from build123d import *

# Parameters (mm, degrees)
SKETCH1_R           = 10
BOSS_EXTRUDE1_DEPTH = 5
BOSS_EXTRUDE3_START = 2
SKETCH3_R           = 12.5
SKETCH3_R_2         = 3.5
SKETCH3_R_3         = 0.95
BOSS_EXTRUDE3_DEPTH = 2


with BuildPart() as part:
    # Sketch1 → Boss-Extrude1 (new body)
    with BuildSketch(Plane.XY):
        with BuildLine():
            Line((-25, 13.756613757), (-25, 11.243386243))
            Line((-25, 11.243386243), (-22.480898871, 11.243386243))
            ThreePointArc((-22.480898871, 11.243386243), (-15.409831059, 8.314454055), (-12.480898871, 1.243386243))
            Line((-12.480898871, 1.243386243), (-12.480898871, 0.690770135))
            ThreePointArc((-12.480898871, 0.690770135), (0, -12.5), (12.480898871, 0.690770135))
            Line((12.480898871, 0.690770135), (12.480898871, 1.243386243))
            ThreePointArc((12.480898871, 1.243386243), (15.409831059, 8.314454055), (22.480898871, 11.243386243))
            Line((22.480898871, 11.243386243), (25, 11.243386243))
            Line((25, 11.243386243), (25, 13.756613757))
            Line((25, 13.756613757), (-25, 13.756613757))
        make_face()
        Circle(SKETCH1_R, mode=Mode.SUBTRACT)
    extrude(amount=BOSS_EXTRUDE1_DEPTH)

    # Sketch3 → Boss-Extrude3 (add)
    with BuildSketch(Plane(origin=(0, 0, 0), x_dir=(-1, 0, 0), z_dir=(0, 0, -1)).offset(BOSS_EXTRUDE3_START)):
        Circle(SKETCH3_R)
        Circle(SKETCH3_R_2, mode=Mode.SUBTRACT)
        with Locations((7.5, 0)):
            Circle(SKETCH3_R_3, mode=Mode.SUBTRACT)
        with Locations((-7.5, 0)):
            Circle(SKETCH3_R_3, mode=Mode.SUBTRACT)
    extrude(amount=-BOSS_EXTRUDE3_DEPTH)


solid = part.part
Here's how the part is built. I have some questions about the finished solid (model axes, mm). A direction names the side the tool comes from. Coordinates: 2 decimals unless noted, no trailing zeros. Order: outer loops, then holes, each group sorted by start corner. A loop starts at its lowest first (then second) coordinate and runs counter-clockwise, first axis right, second up.
Item 1: For faces 1 (the face through (24, 11.243, 2)), 2 (the face through (0, 13, 0)), 3 (the face through (-2.17, -9.76, 2.46)), which set-ups out of +Z, -Z, +X, -X, +Y, -Y let a thin tool reach every point of the face, with its end or its side?
Result sheet:
face 1: +Z, -Z, +X, -Y
face 2: -Z, +Y
face 3: +Z
Item 2: If we section it at A-A on y = 0: List the corners of the cut face in (x, z) for me, plus the area to 3 significant figures.
Result sheet:
outline: (-12.5, -2) - (-8.45, -2) - (-8.45, 0) - (-10, 0) - (-10, 5) - (-12.5, 5) - close; (-6.55, -2) - (-3.5, -2) - (-3.5, 0) - (-6.55, 0) - close; (3.5, -2) - (6.55, -2) - (6.55, 0) - (3.5, 0) - close; (8.45, -2) - (12.5, -2) - (12.5, 5) - (10, 5) - (10, 0) - (8.45, 0) - close
area: 53.4 mm2
Item 3: For P1, Ø1.3, axis at x = -23, z = 2.5, coming from the -Y side; P2, Ø11, axis at x = 0, y = 0, coming from the -Z side; P3, Ø10, axis at x = 3.5, y = -3.5, coming from the +Z side; P4, Ø0.6, axis at y = 1, z = 3, coming from the +X side, each with a flat end and sliding along its axis, tell me the tip position at first contact or that it passes through.
Result sheet:
P1: stops at y = 11.24
P2: stops at z = -2
P3: stops at z = 0
P4: stops at x = 12.48
Item 4: I need wall thicknesses on line 1 (Y direction, x = -7.5, z = -0.7); line 2 (Z direction, x = 14.5, y = 9); line 3 (Y direction, x = 0, z = -1.3). Which ranges of each line are inside material? Lowest first, please.
Result sheet:
line 1: y = -10 to -0.95, 0.95 to 10
line 2: z = 0 to 5
line 3: y = -12.5 to -3.5, 3.5 to 12.5
Item 5: If we section it at D-D on y = 4.25: List the corners of the cut face in (x, z) for me, plus the area to 3 significant figures.
Result sheet:
outline: (-12.94, 0) - (-11.76, 0) - (-11.76, -2) - (11.76, -2) - (11.76, 0) - (12.94, 0) - (12.94, 5) - (9.05, 5) - (9.05, 0) - (-9.05, 0) - (-9.05, 5) - (-12.94, 5) - close
area: 85.9 mm2
Item 6: If we section it at C-C on x = 0: List the corners of the cut face in (y, z) for me.
Result sheet:
outline: (-12.5, -2) - (-3.5, -2) - (-3.5, 0) - (-10, 0) - (-10, 5) - (-12.5, 5) - close; (3.5, -2) - (12.5, -2) - (12.5, 0) - (13.76, 0) - (13.76, 5) - (10, 5) - (10, 0) - (3.5, 0) - close
Item 7: If we mould it in two halves opening along X, with no side actions, what happens to faces 4 (the face through (-6.55, 0.04, -1.01)), 5 (the face through (15.333, 8.236, 2.465)), 6 (the face through (-24, 11.243, 2))? For each: +X half, -X half, draft (parallel to the pull), parting line (faces both ways), or undercut.
Result sheet:
face 4: undercut
face 5: +X half
face 6: draft
Item 8: If we section it at B-B on z = 2.75: List the corners of the cut face in (x, y) for me.
Result sheet:
outline: (-25, 11.24) - (-22.48, 11.24) arc R10 cw to (-12.48, 1.24) - (-12.48, 0.69) arc R12.5 ccw (long way) to (12.48, 0.69) - (12.48, 1.24) arc R10 cw to (22.48, 11.24) - (25, 11.24) - (25, 13.76) - (-25, 13.76) - close; hole circle Ø20 at (0, 0)
